Part model, mm, in its own coordinate system. Face numbers are marked on the shaded views. Round coordinates to 2 decimals unless told otherwise and drop trailing zeros. Loops run counter-clockwise (first coordinate to the right, second up) from the corner with the lowest first, then second, coordinate; pieces in that order, holes last. Notation, with made-up numbers: (14, 8.25) - (66, 8.25) arc R16 ccw to (66, 39.25) - close; hole circle Ø2 at (-14, 53.5). An arc over 180 degrees is marked (long way). Write each question's results on one line, items separated by ' | '. Start each with the question number.
(1) Cut at B-B, the plane z = 62. List the corners of the cut face in (x, y), then the cut area to 3 significant figures.
(2) Cut at A-A, the plane y = 33. List the corners of the cut face in (x, z).
(3) Drill centre lines: L1, parallel to X at y = 34, z = 0; L2, parallel to Y at x = 78, z = -69; L3, parallel to Y at x = -36, z = 16. Where is each one in solid material? Low to high.
(4) Mould opens along X. For the marked faces 1, 2 and 3 say: released by +X, released by -X, zero draft, split by the parting line, or undercut.
(5) Flat gauge pins, fed straight in: P1, Ø5, axis at x = 27, z = -7.5, coming from the -Y side; P2, Ø4, axis at x = 9, y = 5, coming from the +Z side; P3, Ø4, axis at y = 76.5, z = 23, coming from the +X side; P4, Ø10, axis at x = -12.5, y = 43, coming from the +Z side. Where does each tip first touch, or does it go through?
(6) Cut at D-D, the plane x = 5. List the corners of the cut face in (y, z), then the cut area to 3 significant figures.
(7) Cut at C-C, the plane x = 36. List the corners of the cut face in (y, z), then the cut area to 3 significant figures.
from build123d import *

# Parameters (mm, degrees)
SKETCH_2_W               = 46
SKETCH_2_H               = 30
CUT_EXTRUDE_1_DEPTH      = 180.0251379
PATTERN_CIRCULAR_1_COUNT = 3
SKETCH_3_W               = 30
SKETCH_3_H               = 70
CUT_EXTRUDE_2_DEPTH      = 180.0251379


with BuildPart() as part:
    # 草图1 → 旋转1 (revolve)
    with BuildSketch(Plane.XY):
        Polygon((-105, 100), (-100, 100), (-100, 8), (0, 8), (0, 0), (-105, 0), align=None)
    revolve(axis=Axis((0, 100, 0), (0, -1, 0)))

    # 草图2 → 切除-拉伸1 (cut, through all)
    with BuildSketch(Plane.XY):
        with Locations((0, 45)):
            Rectangle(SKETCH_2_W, SKETCH_2_H)
    cut_extrude_1 = extrude(amount=CUT_EXTRUDE_1_DEPTH, mode=Mode.SUBTRACT)

    # 阵列(圆周)1: 切除-拉伸1 ×3 about axis
    pattern_circular_1_axis = Axis((0, 0, 0), (0, 1, 0))
    for i in range(1, PATTERN_CIRCULAR_1_COUNT):
        add(cut_extrude_1.rotate(pattern_circular_1_axis, i * 360 / PATTERN_CIRCULAR_1_COUNT), mode=Mode.SUBTRACT)

    # 草图3 → 切除-拉伸2 (cut, through all)
    with BuildSketch(Plane(origin=(0, 0, 0), x_dir=(1, 0, 0), z_dir=(0, 1, 0))):
        with Locations((35, -45)):
            Rectangle(SKETCH_3_W, SKETCH_3_H)
        with BuildLine():
            Line((-17, -54.8), (-1, -54.8))
            ThreePointArc((-1, -54.8), (0.8, -53), (-1, -51.2))
            Line((-1, -51.2), (-17, -51.2))
            ThreePointArc((-17, -51.2), (-18.8, -53), (-17, -54.8))
        make_face()
        with BuildLine():
            Line((-17, -38.8), (-1, -38.8))
            ThreePointArc((-1, -38.8), (0.8, -37), (-1, -35.2))
            Line((-1, -35.2), (-17, -35.2))
            ThreePointArc((-17, -35.2), (-18.8, -37), (-17, -38.8))
        make_face()
        with BuildLine():
            Line((17, 38.8), (1, 38.8))
            ThreePointArc((1, 38.8), (-0.8, 37), (1, 35.2))
            Line((1, 35.2), (17, 35.2))
            ThreePointArc((17, 35.2), (18.8, 37), (17, 38.8))
        make_face()
        with BuildLine():
            Line((17, 54.8), (1, 54.8))
            ThreePointArc((1, 54.8), (-0.8, 53), (1, 51.2))
            Line((1, 51.2), (17, 51.2))
            ThreePointArc((17, 51.2), (18.8, 53), (17, 54.8))
        make_face()
        with Locations((-35, 45)):
            Rectangle(SKETCH_3_W, SKETCH_3_H)
    extrude(amount=CUT_EXTRUDE_2_DEPTH, mode=Mode.SUBTRACT)


solid = part.part
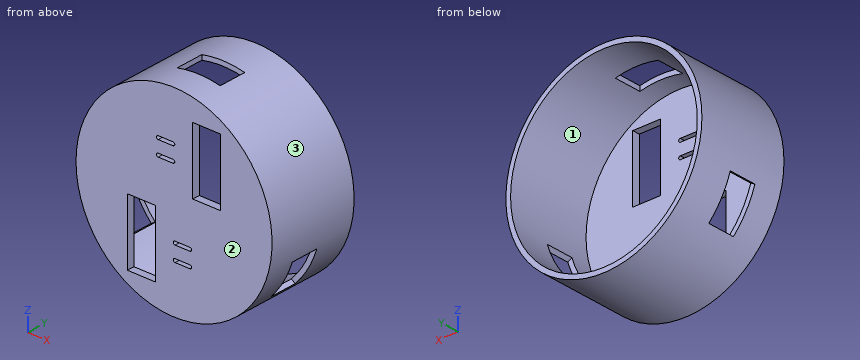
A:
1) outline: (-84.74, 0) - (20, 0) - (20, 8) - (-78.46, 8) - (-78.46, 100) - (-84.74, 100) - close; (50, 0) - (84.74, 0) - (84.74, 100) - (78.46, 100) - (78.46, 8) - (50, 8) - close | area: 2,270 mm2
2) outline: (-100.22, -31.31) - (-95.78, -28.74) arc R100 cw to (-23, 97.32) - (-23, 102.45) arc R105 ccw to start; (-77.22, -71.14) arc R105 ccw to (77.22, -71.14) - (72.78, -68.58) arc R100 cw to (-72.78, -68.58) - close; (23, 97.32) arc R100 cw to (95.78, -28.74) - (100.22, -31.31) arc R105 ccw to (23, 102.45) - close
3) L1: -105 to -100, 100 to 105 | L2: 0 to 30, 60 to 100 | L3: 0 to 8
4) face 1: undercut | face 2: zero draft | face 3: split by the parting line
5) P1: y = 0 | P2: z = 104.77 | P3: x = 102.88 | P4: z = -98.46
6) outline: (0, -104.88) - (100, -104.88) - (100, -99.87) - (8, -99.87) - (8, -54.8) - (0, -54.8) - close; (0, -51.2) - (8, -51.2) - (8, -38.8) - (0, -38.8) - close; (0, -35.2) - (8, -35.2) - (8, 99.87) - (30, 99.87) - (30, 104.88) - (0, 104.88) - close; (60, 99.87) - (100, 99.87) - (100, 104.88) - (60, 104.88) - close | area: 2,390 mm2
7) outline: (0, -98.64) - (100, -98.64) - (100, -93.3) - (8, -93.3) - (8, 10) - (0, 10) - close; (0, 80) - (8, 80) - (8, 93.3) - (100, 93.3) - (100, 98.64) - (0, 98.64) - close | area: 2,000 mm2
